from build123d import *

# Parameters (mm, degrees)
F1_DEPTH      = 1.5875
F2_DEPTH      = 1.5875
F3_DEPTH      = 1.5875
F3_DEPTH_BACK = 1.5875


with BuildPart() as f1:
    # F0 (on Top) → F1 (new body)
    with BuildSketch(Plane.XY):
        with BuildLine():
            Line((-101.5884131193, -18.8973024487), (-89.4398242235, -13.247538358))
            ThreePointArc((-89.4398242235, -13.247538358), (-63.9605427044, -8.860636447), (-38.1898805499, -10.9370918944))
            ThreePointArc((-38.1898805499, -10.9370918944), (-32.4660196125, -12.0949158123), (-26.640561875, -11.6860363632))
            ThreePointArc((-26.640561875, -11.6860363632), (-14.7586255851, -10.8029487579), (-4.7904760577, -17.3295289278))
            Line((-4.7904760577, -17.3295289278), (-2.6797975879, -23.1362432241))
            Line((-2.6797975879, -23.1362432241), (2.6188781485, -24.9024685472))
            Line((2.6188781485, -24.9024685472), (3.3253682777, -20.8401493728))
            add(Edge.make_bspline(
                [(3.8662650694, -18.4174778796), (3.611906377, -19.0656781935), (3.4231723145, -19.8621077155), (3.3253682777, -20.8401493728)],
                knots=[0.9006018819, 0.9006018819, 0.9006018819, 0.9006018819, 1, 1, 1, 1], degree=3))
            ThreePointArc((3.8662650694, -18.4174778796), (9.6420642738, -2.2568424674), (17.1927238868, 13.1546315953))
            add(Edge.make_bspline(
                [(19.2337166518, 14.6902082488), (18.6318591554, 14.4187646386), (17.59365201, 13.7314004824), (17.1927238868, 13.1546315953)],
                knots=[0, 0, 0, 0, 2.5541431294, 2.5541431294, 2.5541431294, 2.5541431294], degree=3))
            add(Edge.make_bspline(
                [(83.2952766221, 17.6661035357), (80.4809135378, 16.6286477767), (74.7370679332, 14.5111030682), (64.3408485466, 15.5369801541), (53.4850420824, 16.9731062249), (39.4603352069, 19.1405437268), (27.191213055, 18.2323443266), (21.8879047106, 15.9122857049), (19.2337166518, 14.6902082488)],
                knots=[0, 0, 0, 0, 0.1519877595, 0.3134001461, 0.4827768067, 0.6751193638, 0.8516699299, 1, 1, 1, 1], degree=3))
            add(Edge.make_bspline(
                [(83.2952766221, 17.6661035357), (75.4343407531, 19.4467237762), (66.8526441437, 21.1255448484), (57.3383793235, 22.663006559)],
                knots=[0.6805820288, 0.6805820288, 0.6805820288, 0.6805820288, 1, 1, 1, 1], degree=3))
            add(Edge.make_bspline(
                [(57.3383793235, 22.663006559), (51.3860041145, 23.5646728097), (39.5545116639, 25.1027234946), (25.1310915838, 23.9086109925), (18.7821781751, 24.0979107297), (10.2035533763, 24.7548514651), (6.1330744065, 25.4)],
                knots=[0, 0, 0, 0, 0.3045684162, 0.5682644154, 0.7491025184, 1, 1, 1, 1], degree=3))
            Line((6.1330744065, 25.4), (1.5553526144, 25.95639154))
            Line((1.5553526144, 25.95639154), (-6.6837654449, 25.4))
            Line((-6.6837654449, 25.4), (-20.9665372968, 25.4))
            Line((-20.9665372968, 25.4), (-73.9454105496, 25.4))
            ThreePointArc((-73.9454105496, 25.4), (-92.1467392312, 23.4934617336), (-109.5579192042, 17.8566128016))
            Line((-109.5579192042, 17.8566128016), (-109.5579192042, -1.152076642))
            Line((-109.5579192042, -1.152076642), (-109.4557195902, -6.2945531681))
            Line((-109.4557195902, -6.2945531681), (-107.5249388814, -15.3543483466))
            Line((-107.5249388814, -15.3543483466), (-101.5884131193, -18.8973024487))
        make_face()
    extrude(amount=F1_DEPTH)

    # F2 (add): a face of the model
    f2_faces = [f1.faces().sort_by_distance(p)[0] for p in [
        (-39.6121775227, 7.2978383867, 0),
    ]]
    extrude(f2_faces, amount=F2_DEPTH)

    # F0 (on Top) → F3 (join, two sides)
    with BuildSketch(Plane.XY) as f3_sk:
        with BuildLine():
            ThreePointArc((17.1927238868, 13.1546315953), (9.6420642738, -2.2568424674), (3.8662650694, -18.4174778796))
            add(Edge.make_bspline(
                [(11.5028988087, -21.510926818), (11.6403456009, -18.4112889852), (10.6938808175, -15.9301904115), (7.0077218043, -15.3266314496), (4.5871981853, -16.580272839), (3.8662650694, -18.4174778796)],
                knots=[0, 0, 0, 0, 0.354240575, 0.6188761258, 0.9006018819, 0.9006018819, 0.9006018819, 0.9006018819], degree=3))
            add(Edge.make_bspline(
                [(61.4279137712, -23.1528356665), (55.5369847146, -23.2709089404), (40.3623363295, -23.3563614522), (16.3717952101, -22.5488794213), (11.5028988087, -21.510926818)],
                knots=[0, 0, 0, 0, 0.4717155518, 1, 1, 1, 1], degree=3))
            add(Edge.make_bspline(
                [(61.4279137712, -23.1528356665), (69.7385266657, -23.0155210755), (95.0642582897, -21.4162605515), (111.9931118186, -10.1613653445), (119.5524930257, -1.1537255666), (123.7895080587, 4.9438558941)],
                knots=[0, 0, 0, 0, 0.3929440031, 0.7004054275, 1, 1, 1, 1], degree=3))
            add(Edge.make_bspline(
                [(123.7895080587, 4.9438558941), (118.1227580639, 7.9880751421), (105.1050021221, 12.2740321559), (89.5844015046, 16.2415221313), (83.2952766221, 17.6661035357)],
                knots=[0, 0, 0, 0, 0.425032366, 0.6805820288, 0.6805820288, 0.6805820288, 0.6805820288], degree=3))
            add(Edge.make_bspline(
                [(83.2952766221, 17.6661035357), (80.4809135378, 16.6286477767), (74.7370679332, 14.5111030682), (64.3408485466, 15.5369801541), (53.4850420824, 16.9731062249), (39.4603352069, 19.1405437268), (27.191213055, 18.2323443266), (21.8879047106, 15.9122857049), (19.2337166518, 14.6902082488)],
                knots=[0, 0, 0, 0, 0.1519877595, 0.3134001461, 0.4827768067, 0.6751193638, 0.8516699299, 1, 1, 1, 1], degree=3))
            add(Edge.make_bspline(
                [(19.2337166518, 14.6902082488), (18.6318591554, 14.4187646386), (17.59365201, 13.7314004824), (17.1927238868, 13.1546315953)],
                knots=[0, 0, 0, 0, 2.5541431294, 2.5541431294, 2.5541431294, 2.5541431294], degree=3))
        make_face()
    extrude(amount=F3_DEPTH)
    extrude(f3_sk.sketch, amount=-F3_DEPTH_BACK)


solid = f1.part
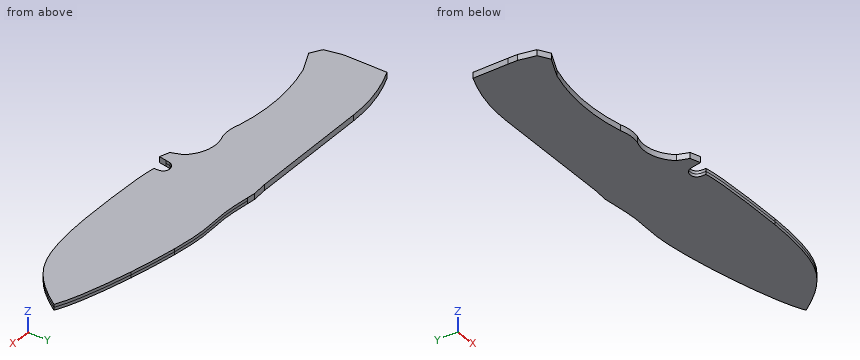
Input: part model. Units: mm. Frame: model coordinates. Coordinates: 2 decimals unless noted, no trailing zeros. Loops run counter-clockwise (first coordinate to the right, second up) from the corner with the lowest first, then second, coordinate; pieces in that order, holes last.
Q1. Cut plane A-A (x = -29). Output: boundary loops of the cut face in (y, z).
Q2. Material intervals for line 1 (Y direction, x = 82.5, z = -1.2); line 2 (X direction, y = 6, z = 1.2); line 3 (X direction, y = -4.5, z = 0.75), sorted ascending.
Q3. Contact query for flat-ended pins moving along their axis: pin 1 (1.5 mm diameter, centred on x = -29, z = 1, fed in from -Y); pin 2 (1.5 mm diameter, centred on x = -4, z = 0, fed in from +Y); pin 3 (1.5 mm diameter, centred on y = -14, z = 0, fed in from -X). Output: stop coordinate, or through.
Working result:
1. outline: (-12.04, -1.59) - (25.4, -1.59) - (25.4, 1.59) - (-12.04, 1.59) - close
2. line 1: y = -21.56 to 17.85
2. line 2: x = -109.56 to 121.7
2. line 3: x = -109.49 to 116.45
3. pin 1: stops at y = -12.1
3. pin 2: stops at y = 25.63
3. pin 3: stops at x = -107.97
